Input: part model. Units: mm. Frame: model coordinates. Coordinates: 2 decimals unless noted, no trailing zeros. Loops run counter-clockwise (first coordinate to the right, second up) from the corner with the lowest first, then second, coordinate; pieces in that order, holes last. Notation, with made-up numbers: (44, 12.5) - (84, 12.5) arc R22 ccw to (84, 48.5) - close; hole circle Ø10 at (-5.75, 81.5). An arc over 180 degrees is marked (long way). Use one line per item in the form item = value.
from build123d import *

# Parameters (mm, degrees)
SWEEP_1_PROFILE_R   = 5
SWEEP_1_PROFILE_R_2 = 4


with BuildPart() as part:
    # 扫描-薄件1: sweep along a path in 草图1
    with BuildLine(Plane.XY) as sweep_1_path:
        Line((78, 30), (78, 20))
        ThreePointArc((78, 20), (75.071067812, 12.928932188), (68, 10))
        Line((68, 10), (0, 10))
        ThreePointArc((0, 10), (-7.071067812, 7.071067812), (-10, 0))
    # 扫描-薄件1 profile (on start of the path) → 扫描-薄件1 (sweep)
    with BuildSketch(Plane(origin=(78, 30, 0), x_dir=(0, 0, -1), z_dir=(0, -1, 0))):
        Circle(SWEEP_1_PROFILE_R)
        Circle(SWEEP_1_PROFILE_R_2, mode=Mode.SUBTRACT)
    sweep(path=sweep_1_path.line)


solid = part.part
Q1. First-contact query: P1, Ø1.5, axis at y = 16, z = -4, coming from the +X side; P2, Ø4, axis at x = 4.5, z = 1.5, coming from the +Y side; P3, Ø2, axis at x = 31.5, y = 7.5, coming from the -Z side. Flat tips, straight axial feed; report the tip coordinate or a pass-through.
Check values:
P1 = 81.24
P2 = 15
P3 = -4.77
Q2. Pull-direction query (X, two-part tool) for faces 1 (the cylindrical face through (33.524, 5.043, 0.651)), 2 (the cylindrical face through (73.12, 24.93, 1.08)), 3 (the cylindrical face through (33.524, 13.905, 0.867)); classes: pulls with the +X half, pulls with the -X half, needs draft (parallel to the pull), parting line crosses it, or undercut.
Check values:
face_1 = needs draft
face_2 = parting line crosses it
face_3 = undercut
Q3. Cut plane A-A, the plane z = 0. Return loops of the section in (x, y), then the cut area to 3 significant figures.
Check values:
outline = (-15, 0) - (-14, 0) arc R14 cw to (0, 14) - (68, 14) arc R6 ccw to (74, 20) - (74, 30) - (73, 30) - (73, 20) arc R5 cw to (68, 15) - (0, 15) arc R15 ccw to start; (-6, 0) - (-5, 0) arc R5 cw to (0, 5) - (68, 5) arc R15 ccw to (83, 20) - (83, 30) - (82, 30) - (82, 20) arc R14 cw to (68, 6) - (0, 6) arc R6 ccw to start
area = 219 mm²
Q4. Ray query, line 1 along Y through (x, z) = (48.5, 0); line 2 along X through (y, z) = (28, 0); line 3 along Z through (x, y) = (20.5, 10). Return the intervals inside material, ascending. Write a range as [from, to].
Check values:
line_1 = [5, 6], [14, 15]
line_2 = [73, 74], [82, 83]
line_3 = [-5, -4], [4, 5]
Q5. Cut plane C-C, the plane y = 24. Return loops of the section in (x, z), then the cut area to 3 significant figures.
Check values:
outline = circle Ø10 at (78, 0); hole circle Ø8 at (78, 0)
area = 28.3 mm²
Q6. Cut plane B-B, the plane x = 53.5. Return loops of the section in (y, z).
Check values:
outline = circle Ø10 at (10, 0); hole circle Ø8 at (10, 0)
